```python
from build123d import *

# Parameters (mm, degrees)
F3_DEPTH        = 20
F4_R            = 5.25
F5_R            = 0.3
F7_D            = 4.4
F7_CSINK_D      = 8.96
F7_CSINK_ANGLE  = 90
F8_DEPTH        = 12.5
F10_D           = 4.4
F10_CSINK_D     = 8.96
F10_CSINK_ANGLE = 90
F11_DEPTH       = 2.5
F12_R           = 3


with BuildPart() as f3:
    # F2 (on Front) → F3 (new body, symmetric)
    with BuildSketch(Plane.XZ):
        with BuildLine():
            ThreePointArc((-2.276188083, 14.2404423798), (-6.1249331198, 3.4778868396), (5.25, 2.357022604))
            ThreePointArc((5.25, 2.357022604), (6.7314560089, 4.6644402004), (7.25, 7.357022604))
            ThreePointArc((7.25, 7.357022604), (4.2461827798, 13.2334527959), (-2.276188083, 14.2404423798))
        make_face()
        with BuildLine():
            ThreePointArc((5.25, 7.357022604), (4.2406721496, 4.261994378), (1.6007810594, 2.357022604))
            ThreePointArc((1.6007810594, 2.357022604), (-4.2406721496, 10.4520508299), (5.25, 7.357022604))
        make_face(mode=Mode.SUBTRACT)
        with BuildLine():
            Line((26.6666666667, -2.642977396), (26.6666666667, 2.357022604))
            Line((26.6666666667, 2.357022604), (7.25, 2.357022604))
            Line((7.25, 2.357022604), (5.25, 2.357022604))
            ThreePointArc((5.25, 2.357022604), (-6.1249331198, 3.4778868396), (-2.276188083, 14.2404423798))
            Line((-2.276188083, 14.2404423798), (-15.3333333333, 9.9227457429))
            Line((-15.3333333333, 9.9227457429), (-15.3333333333, 6.6159764958))
            Line((-15.3333333333, 6.6159764958), (-25.3333333333, 6.6159764958))
            Line((-25.3333333333, 6.6159764958), (-25.3333333333, -2.642977396))
            Line((-25.3333333333, -2.642977396), (26.6666666667, -2.642977396))
        make_face()
        Polygon((-53.3333333333, -2.642977396), (-25.3333333333, -2.642977396), (-25.3333333333, 6.6159764958), align=None)
        Polygon((-15.3333333333, 9.9227457429), (-25.3333333333, 6.6159764958), (-15.3333333333, 6.6159764958), align=None)
    extrude(amount=F3_DEPTH, both=True)

    # F4
    f4_edges = [f3.edges().sort_by_distance(p)[0] for p in [
        (5.25, 0, 2.357023),
    ]]
    fillet(f4_edges, radius=F4_R)

    # F5
    f5_edges = [f3.edges().sort_by_distance(p)[0] for p in [
        (-53.333333, 0, -2.642977),
    ]]
    fillet(f5_edges, radius=F5_R)

    # F7 (through all)
    with Locations(Plane.XY.offset(2.357022604)):
        with Locations((19.5820832083, 12), (19.5820832083, -12)):
            CounterSinkHole(F7_D / 2, F7_CSINK_D / 2, counter_sink_angle=F7_CSINK_ANGLE)

    # F2 (on Front) → F8 (cut, symmetric)
    with BuildSketch(Plane.XZ):
        Polygon((-15.3333333333, 9.9227457429), (-25.3333333333, 6.6159764958), (-15.3333333333, 6.6159764958), align=None)
    extrude(amount=F8_DEPTH, both=True, mode=Mode.SUBTRACT)

    # F10 (through all)
    with Locations(Plane.XY.offset(6.6159764958)):
        with Locations((-20.3333333333, -7.5), (-20.3333333333, 7.5)):
            CounterSinkHole(F10_D / 2, F10_CSINK_D / 2, counter_sink_angle=F10_CSINK_ANGLE)

    # F2 (on Front) → F11 (join, symmetric)
    with BuildSketch(Plane.XZ):
        Polygon((-15.3333333333, 9.9227457429), (-25.3333333333, 6.6159764958), (-15.3333333333, 6.6159764958), align=None)
    extrude(amount=F11_DEPTH, both=True)

    # F12
    f12_edges = [f3.edges().sort_by_distance(p)[0] for p in [
        (26.666667, -20, -0.142977),
        (26.666667, 20, -0.142977),
    ]]
    fillet(f12_edges, radius=F12_R)


solid = f3.part
```
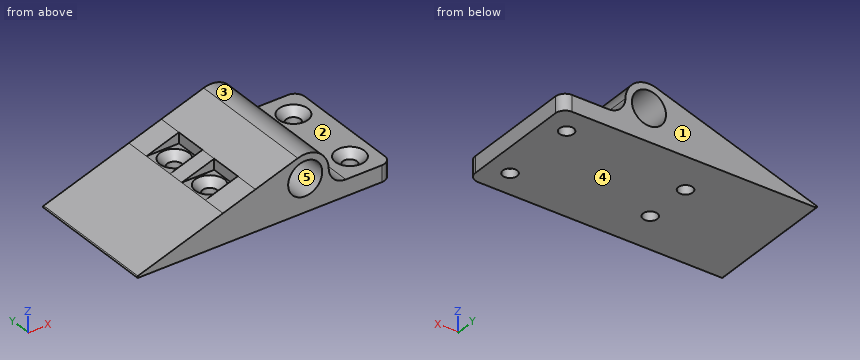
Part model, mm, in its own coordinate system. Face numbers are marked on the shaded views. A direction names the side the tool comes from. Give positions to 0.01 mm unless a question says otherwise; leave off trailing zeros. Order: outer loops, then holes, each group sorted by start corner. A loop starts at its lowest first (then second) coordinate and runs counter-clockwise, first axis right, second up. Notation, with made-up numbers: M 39.5,6.5 L 72.5,6.5 A21 cw 72.5,14.5 Z; hole C -33,47.25 d11. An arc over 180 degrees is marked long. Use a Markdown table: item, result. Add a question column.
(1) Saw through at C-C, the plane z = 1. Give the cut face in (x, y).
(2) Saw through at D-D, the plane x = -12. Give the cut face in (y, z) (3 decimals), and give its area (3 significant figures).
(3) Mould opens along X. For the marked faces 3, 4 and 5 say: +X half, -X half, draft (parallel to the pull), parting line (faces both ways), or undercut.
(4) Saw through at A-A, the plane z = 11.25. Give the cut face in (x, y), and give its area (3 significant figures).
(5) Saw through at B-B, the plane x = 14. Give the cut face in (y, z), and give its area (3 significant figures).
(6) Drop flat-ended pins along their axis: P1, Ø3.5, axis at y = 9, z = 8.5, coming from the -X side; P2, Ø1.5, axis at y = -1, z = 5, coming from the +X side; P3, Ø11, axis at x = -19, y = 9.5, coming from the +Z side; P4, Ø5, axis at x = -20.33, y = -7.5, coming from the -Z side. Give the stop position or say it passes through.
(7) 3-axis set-ups, long thin cutter, end or side, ignore diameter. For the marked faces 1 and 2: which of +Z, -Z, +X, -X, +Y, -Y reach the whole face in a straight line?
(8) Probe line 1 along Z through (x, y) = (0, -3); line 2 along Y through (x, z) = (19.5, 1); line 3 along X through (y, z) = (5, 7.5). List the from-to ranges inside material, lowest first. Write a range as [from, to].
Answer key:
| question | item | result |
|---|---|---|
| 1 | outline | M -42.32,-20 L 23.67,-20 A3 ccw 26.67,-17 L 26.67,17 A3 ccw 23.67,20 L -42.32,20 Z; hole C -20.33,-7.5 d4.4; hole C -20.33,7.5 d4.4; hole C 19.58,-12 d6.25; hole C 19.58,12 d6.25 |
| 2 | outline | M -20,-2.643 L 20,-2.643 L 20,11.025 L -20,11.025 Z |
| 2 | area | 547 mm^2 |
| 3 | face 3 | parting line |
| 3 | face 4 | draft |
| 3 | face 5 | undercut |
| 4 | outline | M -11.32,-20 L -3.52,-20 L -3.52,20 L -11.32,20 Z; M 3.52,-20 L 6.12,-20 L 6.12,20 L 3.52,20 Z |
| 4 | area | 416 mm^2 |
| 5 | outline | M -20,-2.64 L 20,-2.64 L 20,2.36 L -20,2.36 Z |
| 5 | area | 200 mm^2 |
| 6 | P1 | x = -15.33 |
| 6 | P2 | x = 8.46 |
| 6 | P3 | z = 10.53 |
| 6 | P4 | z = -2.64 |
| 7 | face 1 | +Z, -Z, +X, -X, +Y |
| 7 | face 2 | +Z, +X, +Y, -Y |
| 8 | line 1 | [-2.64, 2.11], [12.61, 14.61] |
| 8 | line 2 | [-20, -15.12], [-8.88, 8.88], [15.12, 20] |
| 8 | line 3 | [-15.33, -5.25], [5.25, 7.25] |
